Part model, mm, in its own coordinate system. Face numbers are marked on the shaded views. A direction names the side the tool comes from. Give positions to 0.01 mm unless a question says otherwise; leave off trailing zeros. Order: outer loops, then holes, each group sorted by start corner. A loop starts at its lowest first (then second) coordinate and runs counter-clockwise, first axis right, second up. Notation, with made-up numbers: M 78.25,-27.75 L 107.25,-27.75 A11 ccw 107.25,-6.75 Z; hole C 31.25,-28.5 d6. An arc over 180 degrees is marked long. Write each question's results on one line, items separated by ' | '. Start each with the question number.
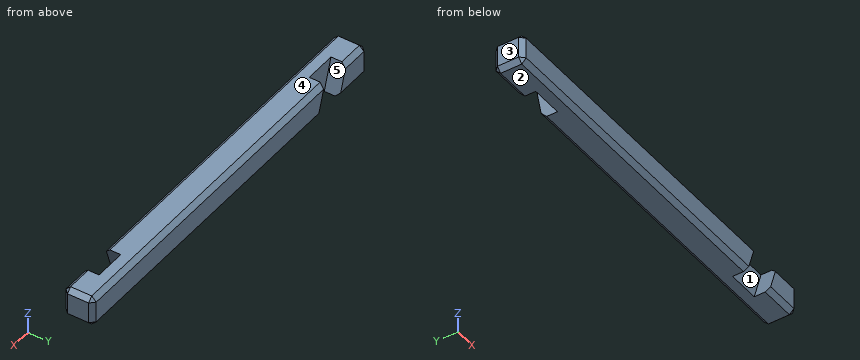
from build123d import *

# Parameters (mm, degrees)
F1_DEPTH = 10
F3_DEPTH = 4.9
F5_DEPTH = 4.9
F6_SIZE  = 1.5


with BuildPart() as f1:
    # F0 (on Front) → F1 (new body)
    with BuildSketch(Plane.XZ):
        Polygon((-60.0217013935, 10), (-60.0217013935, 0), (-46.7717013935, 0), (-50.0208983558, 10), align=None)
    extrude(amount=F1_DEPTH)



with BuildPart() as f1b:
    # F0 (on Front) → F1, piece 2 (new body)
    with BuildSketch(Plane.XZ):
        Polygon((-39.5058983558, 10), (-36.2567013935, 0), (48.7149046818, 0), (51.9641016442, 10), align=None)
    extrude(amount=F1_DEPTH)



with BuildPart() as f1c:
    # F0 (on Front) → F1, piece 3 (new body)
    with BuildSketch(Plane.XZ):
        Polygon((62.4791016442, 10), (59.2299046818, 0), (72.4799046818, 0), (72.4799046818, 10), align=None)
    extrude(amount=F1_DEPTH)


with BuildPart() as f1b_1:
    add(f1b.part)

    add(f1c.part)  # F3 merges F1c
    # F2 (on face) → F3 (join)
    with BuildSketch(Plane(origin=(0, 0, 0), x_dir=(-1, 0, 0), z_dir=(0, 1, 0))):
        Polygon((-51.9641016442, 10), (-62.4791016442, 10), (-59.2299046818, 0), (-48.7149046818, 0), align=None)
    extrude(amount=-F3_DEPTH)


with BuildPart() as f1_1:
    add(f1.part)

    add(f1b_1.part)  # F5 merges F1b
    # F4 (on face) → F5 (join)
    with BuildSketch(Plane.XZ.offset(10)):
        Polygon((-39.5058983558, 10), (-50.0208983558, 10), (-46.7717013935, 0), (-36.2567013935, 0), align=None)
    extrude(amount=-F5_DEPTH)

    # F6
    f6_edges = [f1_1.edges().sort_by_distance(p)[0] for p in [
        (-60.021701, -5, 10),
        (-60.021701, -5, 0),
        (-60.021701, 0, 5),
        (-60.021701, -10, 5),
        (-55.0213, 0, 10),
        (-53.396701, 0, 0),
        (-5.653398, -10, 0),
        (-4.0288, -10, 10),
        (18.111602, 0, 0),
        (65.854905, -10, 0),
        (67.479503, -10, 10),
        (72.479905, -10, 5),
        (72.479905, -5, 0),
        (72.479905, 0, 5),
        (72.479905, -5, 10),
        (16.487003, 0, 10),
    ]]
    chamfer(f6_edges, length=F6_SIZE)


solid = f1_1.part
(1) Saw through at C-C on z = 3.5. Give the cut face in (x, y).
(2) Tool access for the marked faces 4 and 5: list every direction of +Z, -Z, +X, -X, +Y, -Y with a clear straight run to the whole face (end or side of a thin tool).
(3) Drop flat-ended pins along their axis: P1, Ø3, axis at x = 52.5, z = 6, coming from the -Y side; P2, Ø2, axis at x = -11.5, z = 9, coming from the +Y side. Give the stop position or say it passes through.
(4) Pull direction X, two halves, no side cores. Call the marked faces 1, 2 and 3: +X half, -X half, draft (parallel to the pull), parting line (faces both ways), or undercut.
(5) Saw through at B-B on x = -32. Give the cut face in (y, z), plus the area to 3 significant figures.
(6) Probe L1, parallel to X at y = -2, z = 3; L2, parallel to X at y = -7.75, z = 9.5; L3, parallel to Z at x = 38.5, y = -9.5. List the from-to ranges inside material, lowest first.
(7) Saw through at A-A on y = -7. Give the cut face in (x, z), plus the area to 3 significant figures.
(8) Saw through at D-D on x = 58. Give the cut face in (y, z), plus the area to 4 significant figures.
Taken from the geometry:
1) outline: M -60.02,-8.5 L -58.52,-10 L 49.85,-10 L 49.85,-4.9 L 60.37,-4.9 L 60.37,-10 L 70.98,-10 L 72.48,-8.5 L 72.48,-1.5 L 70.98,0 L -37.39,0 L -37.39,-5.1 L -47.91,-5.1 L -47.91,0 L -58.52,0 L -60.02,-1.5 Z
2) face 4: +Z, +X, -X, +Y, -Y | face 5: +Z, +Y
3) P1: stops at y = -4.9 | P2: stops at y = 0
4) face 1: undercut | face 2: draft | face 3: -X half
5) outline: M -10,1.5 L -8.5,0 L -1.5,0 L 0,1.5 L 0,8.5 L -1.5,10 L -8.5,10 L -10,8.5 Z | area: 95.5 mm²
6) L1: x = -60.02 to -47.75, -37.23 to 72.48 | L2: x = -59.02 to 51.8, 62.32 to 71.48 | L3: z = 1 to 9
7) outline: M -60.02,1.5 L -58.52,0 L 48.71,0 L 51.96,10 L -58.52,10 L -60.02,8.5 Z; M 59.23,0 L 70.98,0 L 72.48,1.5 L 72.48,8.5 L 70.98,10 L 62.48,10 Z | area: 1,220 mm²
8) outline: M -4.9,0 L -1.5,0 L 0,1.5 L 0,8.5 L -1.5,10 L -4.9,10 Z | area: 46.75 mm²
